For this review, take the finished solid that the model builds, in its own axes (mm). A direction names the side the tool comes from. Give positions to 0.01 mm unless a question says otherwise; leave off trailing zeros. Loops run counter-clockwise (first coordinate to the right, second up) from the corner with the lowest first, then second, coordinate; pieces in that order, holes last.
```python
from build123d import *

# Parameters (mm, degrees)
F0_W     = 101.6
F0_H     = 50.8
F1_DEPTH = 25.4
F2_W     = 50.8
F2_H     = 25.4
F3_DEPTH = 12.7
F4_W     = 25.4
F4_H     = 11.0103109196
F5_DEPTH = 19.05


with BuildPart() as f1:
    # F0 (on Front) → F1 (new body)
    with BuildSketch(Plane.XZ):
        Rectangle(F0_W, F0_H)
    extrude(amount=F1_DEPTH)

    # F2 (on face) → F3 (cut)
    with BuildSketch(Plane.XY.offset(25.4)):
        with Locations((0, -12.7)):
            Rectangle(F2_W, F2_H)
    extrude(amount=-F3_DEPTH, mode=Mode.SUBTRACT)

    # F4 (on face) → F5 (cut)
    with BuildSketch(Plane.YZ.offset(50.8)):
        with Locations((-12.7, -19.8948445402)):
            Rectangle(F4_W, F4_H)
    extrude(amount=-F5_DEPTH, mode=Mode.SUBTRACT)


solid = f1.part
```
Item 1: Clearance check with flat-ended pins moving along their axes: pin 1 Ø8 at (x, y) = (9, -10.5) entering from +Z; pin 2 Ø9 at (y, z) = (-8, -20) entering from +X; pin 3 Ø4 at (x, y) = (37, -20) entering from -Z. State where each tip first meets the part, or that it passes through.
Answer:
pin 1: stops at z = 12.7
pin 2: stops at x = 31.75
pin 3: stops at z = -14.39
Item 2: Take a section at A-A on z = 22.5. Give the boundary of the cut face in (x, y).
Answer:
outline: (-50.8, -25.4) - (-25.4, -25.4) - (-25.4, 0) - (-50.8, 0) - close; (25.4, -25.4) - (50.8, -25.4) - (50.8, 0) - (25.4, 0) - close
Item 3: Take a section at D-D on z = -18. Give the boundary of the cut face in (x, y), and give its area (3 significant figures).
Answer:
outline: (-50.8, -25.4) - (31.75, -25.4) - (31.75, 0) - (-50.8, 0) - close
area: 2,100 mm2
Item 4: Take a section at C-C on x = 40. Give the boundary of the cut face in (y, z).
Answer:
outline: (-25.4, -14.39) - (0, -14.39) - (0, 25.4) - (-25.4, 25.4) - close
Item 5: Tool access review of faces 1 (the flat face through (31.75, -13, -20)), 2 (the flat face through (-1, -25.4, 0)), 3 (the flat face through (25.4, -13, 19)): name each direction out of +Z, -Z, +X, -X, +Y, -Y from which nothing blocks a thin tool from reaching the whole face with its end or side.
Answer:
face 1: -Z, +X, +Y, -Y
face 2: +Z, -Z, +X, -X, -Y
face 3: +Z, +Y, -Y
Item 6: Take a section at B-B on y = -5. Give the boundary of the cut face in (x, z), and give its area (3 significant figures).
Answer:
outline: (-50.8, -25.4) - (31.75, -25.4) - (31.75, -14.39) - (50.8, -14.39) - (50.8, 25.4) - (25.4, 25.4) - (25.4, 12.7) - (-25.4, 12.7) - (-25.4, 25.4) - (-50.8, 25.4) - close
area: 4,310 mm2
Item 7: For L1, parallel to X at y = -18.25, z = 19; L2, parallel to X at y = -16.5, z = -18.5; L3, parallel to Z at x = 3.5, y = -8.25, list the stretches that pass through material, from the lowest coordinate up.
Answer:
L1: x = -50.8 to -25.4, 25.4 to 50.8
L2: x = -50.8 to 31.75
L3: z = -25.4 to 12.7
